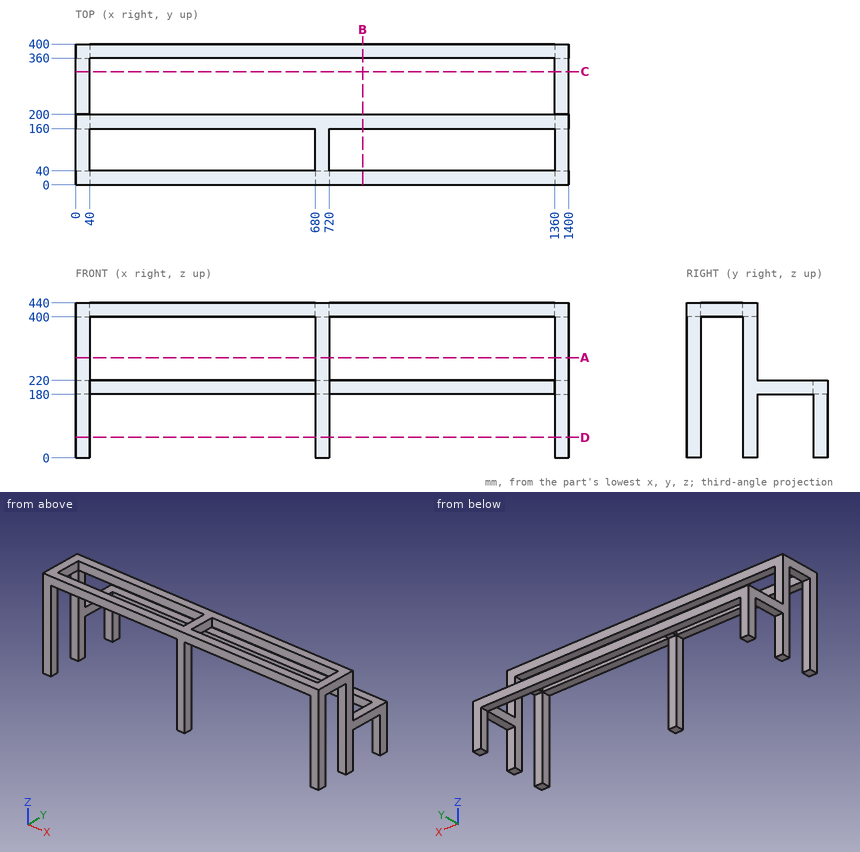
Can you work these out from the drawing? Everything is in mm from the part's minimum corner. Give positions to 0.01 mm unless a question says otherwise; leave off trailing zeros. Loops run counter-clockwise (first coordinate to the right, second up) from the corner with the lowest first, then second, coordinate; pieces in that order, holes last. Notation, with made-up numbers: (57, 41) -> (102, 41) arc R21 ccw to (102, 79) -> close; hole circle Ø1 at (-12.75, 12). An arc over 180 degrees is marked (long way). Return JSON: item names as keys, results as strings.
Item 1: If we section it at A-A on z = 284.5: List the corners of the cut face in (x, y) for me, plus the area to 3 significant figures.
Geometry results:
{"outline": "(0, 0) -> (40, 0) -> (40, 40) -> (0, 40) -> close; (0, 160) -> (40, 160) -> (40, 200) -> (0, 200) -> close; (680, 0) -> (720, 0) -> (720, 40) -> (680, 40) -> close; (1360, 0) -> (1400, 0) -> (1400, 40) -> (1360, 40) -> close; (1360, 160) -> (1400, 160) -> (1400, 200) -> (1360, 200) -> close", "area": "8,000 mm²"}
Item 2: If we section it at D-D on z = 58: List the corners of the cut face in (x, y) for me.
Geometry results:
{"outline": "(0, 0) -> (40, 0) -> (40, 40) -> (0, 40) -> close; (0, 160) -> (40, 160) -> (40, 200) -> (0, 200) -> close; (0, 360) -> (40, 360) -> (40, 400) -> (0, 400) -> close; (680, 0) -> (720, 0) -> (720, 40) -> (680, 40) -> close; (1360, 0) -> (1400, 0) -> (1400, 40) -> (1360, 40) -> close; (1360, 160) -> (1400, 160) -> (1400, 200) -> (1360, 200) -> close; (1360, 360) -> (1400, 360) -> (1400, 400) -> (1360, 400) -> close"}
Item 3: If we section it at C-C on y = 321.5: List the corners of the cut face in (x, z) for me, plus the area to 3 significant figures.
Geometry results:
{"outline": "(0, 180) -> (40, 180) -> (40, 220) -> (0, 220) -> close; (1360, 180) -> (1400, 180) -> (1400, 220) -> (1360, 220) -> close", "area": "3,200 mm²"}
Item 4: If we section it at B-B on x = 815.5: List the corners of the cut face in (y, z) for me, plus the area to 3 significant figures.
Geometry results:
{"outline": "(0, 400) -> (40, 400) -> (40, 440) -> (0, 440) -> close; (160, 400) -> (200, 400) -> (200, 440) -> (160, 440) -> close; (360, 180) -> (400, 180) -> (400, 220) -> (360, 220) -> close", "area": "4,800 mm²"}
Item 5: I need wall thicknesses on L1, parallel to X at y = 194, z = 37; L2, parallel to X at y = 21.5, z = 328; L3, parallel to Z at x = 1227, y = 191.5. Which ranges of each line are inside material? Lowest first, please. Write a range as from..to.
Geometry results:
{"L1": "x = 0..40, 1360..1400", "L2": "x = 0..40, 680..720, 1360..1400", "L3": "z = 400..440"}
Item 6: I'm going to push flat-ended pins straight in: pin 1 (4 mm diameter, centred on y = 157, z = 166, fed in from +X); pin 2 (12 mm diameter, centred on x = 15.5, y = 272.5, fed in from -Z). Where does each tip first touch, or does it pass through?
Geometry results:
{"pin 1": "passes through", "pin 2": "stops at z = 180"}
